The model under review builds one solid part; all positions refer to its coordinate system, in mm. Round coordinates to 2 decimals unless told otherwise and drop trailing zeros.
1) Clearance check with a flat-ended pin moving along its axis: P1, Ø3, axis at x = 10, y = 10, coming from the +Z side. State where the tip first meets the part, or that it passes through.
2) To check wall thickness, follow L1, parallel to X at y = 10, z = 7.75; L2, parallel to Y at x = 5, z = 44. State the ranges of each line that lie inside material, in increasing order.
3) Consider section A-A (x = 10). Give the number of separate pieces and of enclosed holes in the cut face, then the cut area to 3 significant figures.
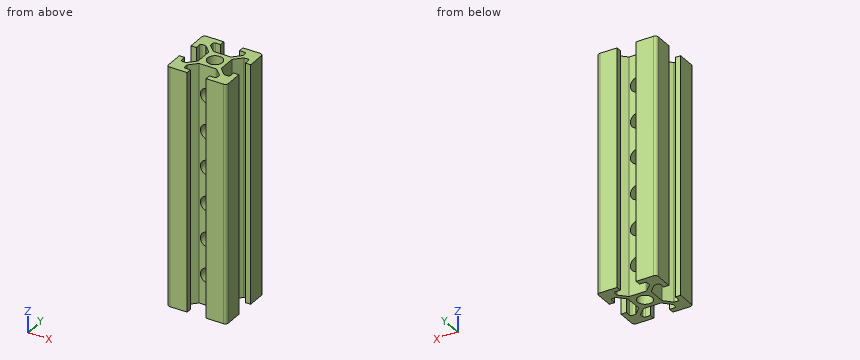
from build123d import *

# Parameters (mm, degrees)
SKETCH1_R           = 2.5
BOSS_EXTRUDE1_DEPTH = 80
FILLET1_R           = 1
FILLET2_R           = 0.5
FILLET3_R           = 0.5
FILLET4_R           = 0.5
FILLET5_R           = 0.5
SKETCH2_R           = 2.5
CUT_EXTRUDE1_DEPTH  = 8


with BuildPart() as part:
    # Sketch1 → Boss-Extrude1 (new body)
    with BuildSketch(Plane.XY):
        Polygon((13.2, 0), (13.2, 1.8), (15.45, 1.8), (15.45, 3.6), (12.95, 6.1), (7.05, 6.1), (4.55, 3.6), (4.55, 1.8), (6.8, 1.8), (6.8, 0), (0, 0), (0, 6.8), (1.8, 6.8), (1.8, 4.55), (3.6, 4.55), (6.1, 7.05), (6.1, 12.95), (3.6, 15.45), (1.8, 15.45), (1.8, 13.2), (0, 13.2), (0, 20), (6.8, 20), (6.8, 18.2), (4.55, 18.2), (4.55, 16.4), (7.05, 13.9), (12.95, 13.9), (15.45, 16.4), (15.45, 18.2), (13.2, 18.2), (13.2, 20), (20, 20), (20, 13.2), (18.2, 13.2), (18.2, 15.45), (16.4, 15.45), (13.9, 12.95), (13.9, 7.05), (16.4, 4.55), (18.2, 4.55), (18.2, 6.8), (20, 6.8), (20, 0), align=None)
        with Locations((10, 10)):
            Circle(SKETCH1_R, mode=Mode.SUBTRACT)
    extrude(amount=BOSS_EXTRUDE1_DEPTH)

    # Fillet1
    fillet1_edges = [part.edges().sort_by_distance(p)[0] for p in [
        (0, 0, 40),
        (0, 20, 40),
        (20, 20, 40),
        (20, 0, 40),
    ]]
    fillet(fillet1_edges, radius=FILLET1_R)

    # Fillet2
    fillet2_edges = [part.edges().sort_by_distance(p)[0] for p in [
        (4.55, 18.2, 40),
        (4.55, 16.4, 40),
        (7.05, 13.9, 40),
        (12.95, 13.9, 40),
        (15.45, 16.4, 40),
        (15.45, 18.2, 40),
    ]]
    fillet(fillet2_edges, radius=FILLET2_R)

    # Fillet3
    fillet3_edges = [part.edges().sort_by_distance(p)[0] for p in [
        (18.2, 15.45, 40),
        (16.4, 15.45, 40),
        (13.9, 12.95, 40),
        (13.9, 7.05, 40),
        (16.4, 4.55, 40),
        (18.2, 4.55, 40),
    ]]
    fillet(fillet3_edges, radius=FILLET3_R)

    # Fillet4
    fillet4_edges = [part.edges().sort_by_distance(p)[0] for p in [
        (1.8, 4.55, 40),
        (3.6, 4.55, 40),
        (6.1, 7.05, 40),
        (6.1, 12.95, 40),
        (3.6, 15.45, 40),
        (1.8, 15.45, 40),
    ]]
    fillet(fillet4_edges, radius=FILLET4_R)

    # Fillet5
    fillet5_edges = [part.edges().sort_by_distance(p)[0] for p in [
        (15.45, 1.8, 40),
        (15.45, 3.6, 40),
        (12.95, 6.1, 40),
        (7.05, 6.1, 40),
        (4.55, 3.6, 40),
        (4.55, 1.8, 40),
    ]]
    fillet(fillet5_edges, radius=FILLET5_R)

    # Sketch2 → Cut-Extrude1 (cut)
    with BuildSketch(Plane(origin=(0, 13.9, 0), x_dir=(1, 0, 0), z_dir=(0, 1, 0))):
        with Locations((10, -58)):
            Circle(SKETCH2_R)
        with Locations((10, -70)):
            Circle(SKETCH2_R)
        with Locations((10, -34)):
            Circle(SKETCH2_R)
        with Locations((10, -46)):
            Circle(SKETCH2_R)
        with Locations((10, -22)):
            Circle(SKETCH2_R)
        with Locations((10, -10)):
            Circle(SKETCH2_R)
    extrude(amount=-CUT_EXTRUDE1_DEPTH, mode=Mode.SUBTRACT)


solid = part.part
Answer below:
1. P1: passes through
2. L1: x = 6.1 to 7.5, 12.5 to 13.9
2. L2: y = 0 to 1.8, 4.05 to 5.95, 14.05 to 15.95, 18.2 to 20
3. separate pieces: 14
3. enclosed holes: 0
3. area: 140 mm2
